```python
from build123d import *

# Parameters (mm, degrees)
F0_W     = 50
F0_H     = 60
F1_DEPTH = 40
F3_START = -50
F2_R     = 5
F3_DEPTH = 400


with BuildPart() as f1:
    # F0 (on Top) → F1 (new body)
    with BuildSketch(Plane.XY):
        with Locations((-125, -30)):
            Rectangle(F0_W, F0_H)
    extrude(amount=F1_DEPTH)



with BuildPart() as f1b:
    # F0 (on Top) → F1, piece 2 (new body)
    with BuildSketch(Plane.XY):
        with Locations((325, -30)):
            Rectangle(F0_W, F0_H)
    extrude(amount=F1_DEPTH)


with BuildPart() as f1_1:
    add(f1.part)

    add(f1b.part)  # F3 merges F1b
    # F2 (on face) → F3 (join)
    with BuildSketch(Plane.YZ.offset(350).offset(F3_START)):
        with Locations((-15, 20)):
            Circle(F2_R)
    extrude(amount=-F3_DEPTH)


solid = f1_1.part
```
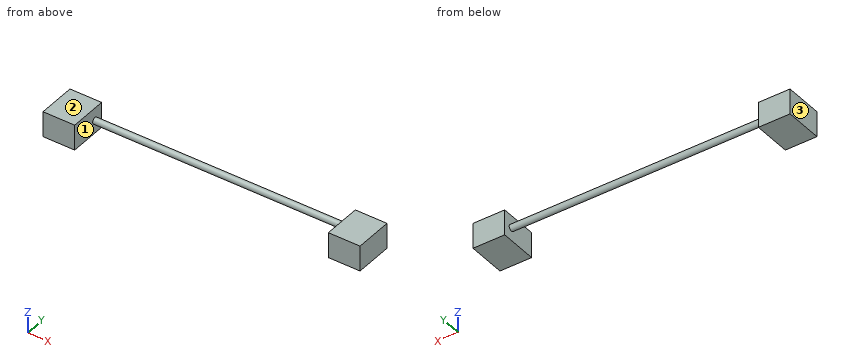
Design review of the part built by this model. Coordinates are the model's own, in mm. Face numbers are marked on the shaded views. Coordinates: 2 decimals unless noted, no trailing zeros. Loops run counter-clockwise (first coordinate to the right, second up) from the corner with the lowest first, then second, coordinate; pieces in that order, holes last. Notation, with made-up numbers: M 70.5,-5 L 80.5,-5 A35 cw 80.5,30 Z; hole C -17.5,58 d10. An arc over 180 degrees is marked long. One line per question, with ' | ' between items.
(1) For pin 1 Ø6 at (x, z) = (144, 16) entering from -Y; pin 2 Ø5 at (x, z) = (288.5, 21.5) entering from +Y, all flat-tipped, find the tip position at first contact; note any pin that passes through.
Filled in:
pin 1: stops at y = -19.9 | pin 2: stops at y = -10
(2) We need section C-C (x = -70.5). Give the boundary of the cut face in (y, z).
Filled in:
outline: C -15,20 d10
(3) We need section A-A (y = -31). Give the boundary of the cut face in (x, z).
Filled in:
outline: M -150,0 L -100,0 L -100,40 L -150,40 Z; M 300,0 L 350,0 L 350,40 L 300,40 Z
(4) We need section B-B (z = 20). Give the boundary of the cut face in (x, y), and give its area (3 significant figures).
Filled in:
outline: M -150,-60 L -100,-60 L -100,-20 L 300,-20 L 300,-60 L 350,-60 L 350,0 L 300,0 L 300,-10 L -100,-10 L -100,0 L -150,0 Z | area: 10,000 mm^2
(5) Draft analysis for pull direction X (two halves, no side actions). For the marked faces 1, 2 and 3, state which applies: released by +X, released by -X, zero draft, split by the parting line, or undercut.
Filled in:
face 1: undercut | face 2: zero draft | face 3: released by -X
(6) Wall thickness on probe 1 along X at (y, z) = (-38, 24); probe 2 along Y at (x, z) = (149.5, 19); probe 3 along Y at (x, z) = (118, 18): over which ranges is each line inside the solid? List them lowest first.
Filled in:
probe 1: x = -150 to -100, 300 to 350 | probe 2: y = -19.9 to -10.1 | probe 3: y = -19.58 to -10.42
